```python
from build123d import *

# Parameters (mm, degrees)
BASE_FLANGE1_DEPTH           = 0.91186
F_2_5MM_DOWEL_HOLE1_D        = 2.5
EDGE_FLANGE1_STRIP_W         = 6.18744
EDGE_FLANGE1_STRIP_H         = 0.91186
EDGE_FLANGE1_STRIP_CUT_DEPTH = 82.55
EDGE_FLANGE1_DEPTH           = 82.55


# Sheet-metal steps are written as plain solids
with BuildPart() as part:
    # Sketch1 → Base-Flange1 (new body)
    with BuildSketch(Plane(origin=(0, 0, 0), x_dir=(1, 0, 0), z_dir=(0, 1, 0))):
        Polygon((0, -24.82463), (0, -48.018817445), (12.7, -48.018817445), (12.7, -37.52463), (69.85, -37.52463), (69.85, -48.018817445), (82.55, -48.018817445), (82.55, -24.82463), align=None)
    extrude(amount=-BASE_FLANGE1_DEPTH)

    # Ø2.5mm Dowel Hole1 (through all)
    with Locations(Plane(origin=(0, -0.91186, 0), x_dir=(-1, 0, 0), z_dir=(0, -1, 0))):
        with Locations((-65.76314, -27.56213), (-16.78686, -27.56213)):
            Hole(F_2_5MM_DOWEL_HOLE1_D / 2)

    # Edge-Flange1 strip (across the edge) → Edge-Flange1 strip cut (cut)
    with BuildSketch(Plane(origin=(82.55, 0, 24.82463), x_dir=(0, 0, 1), z_dir=(-1, 0, 0))):
        with Locations((-1.82372, -0.45593)):
            Rectangle(EDGE_FLANGE1_STRIP_W, EDGE_FLANGE1_STRIP_H)
    extrude(amount=EDGE_FLANGE1_STRIP_CUT_DEPTH, mode=Mode.SUBTRACT)

    # Edge-Flange1 section (across the edge) → Edge-Flange1 (add)
    with BuildSketch(Plane(origin=(82.55, 0, 24.82463), x_dir=(0, 0, 1), z_dir=(-1, 0, 0))):
        with BuildLine():
            Line((-0.91186, 1.27), (-0.91186, 5.43814))
            Line((-0.91186, 5.43814), (0, 5.43814))
            Line((0, 5.43814), (0, 1.27))
            ThreePointArc((0, 1.27), (0.371974388, 0.371974388), (1.27, 0))
            Line((1.27, 0), (1.27, -0.91186))
            ThreePointArc((1.27, -0.91186), (-0.272808002, -0.272808002), (-0.91186, 1.27))
        make_face()
    extrude(amount=EDGE_FLANGE1_DEPTH)


solid = part.part
```
Input: part model. Units: mm. Frame: model coordinates. A direction names the side the tool comes from. Give positions to 0.01 mm unless a question says otherwise; leave off trailing zeros. Order: outer loops, then holes, each group sorted by start corner. A loop starts at its lowest first (then second) coordinate and runs counter-clockwise, first axis right, second up. Notation, with made-up numbers: (18, 20.25) - (46, 20.25) arc R20 ccw to (46, 32.25) - close; hole circle Ø7 at (77, -14). An arc over 180 degrees is marked (long way). Put each result on its own line as item: value.
Item 1: Access query for faces 4 (the flat face through (41, 0, 34)), 5 (the flat face through (82.55, -0.3, 34.2)). Directions: +Z, -Z, +X, -X, +Y, -Y. A direction counts if a zero-diameter tool reaches every point of the face in a straight line with its end or side. Return the directions, or none.
Found:
face 4: +Z, +X, -X, +Y
face 5: +Z, -Z, +X, +Y, -Y
Item 2: Contact query for flat-ended pins moving along their axis: pin 1 (1.3 mm diameter, centred on x = 56, y = 3.5, fed in from +Z); pin 2 (2 mm diameter, centred on x = 65.76, z = 27.56, fed in from -Y); pin 3 (3 mm diameter, centred on x = 16.79, z = 27.56, fed in from +Y); pin 4 (0.5 mm diameter, centred on x = 30, y = -0.5, fed in from +Z). Output: stop coordinate, or through.
Found:
pin 1: stops at z = 24.82
pin 2: passes through
pin 3: stops at y = 0
pin 4: stops at z = 37.52
Item 3: Section query D-D, the plane z = 35.25. Return loops of the section in (x, y).
Found:
outline: (0, -0.91) - (82.55, -0.91) - (82.55, 0) - (0, 0) - close
Item 4: Ray query, L1, parallel to Z at x = 28, y = 4; L2, parallel to X at y = -0.5, z = 44.5; L3, parallel to Y at x = 76, z = 26.25. Return the intervals inside material, ascending. Write a range as from..to.
Found:
L1: z = 23.91..24.82
L2: x = 0..12.7, 69.85..82.55
L3: y = -0.91..0
Item 5: Section query A-A, the plane z = 42. Return loops of the section in (x, y), then the cut area to 3 significant figures.
Found:
outline: (0, -0.91) - (12.7, -0.91) - (12.7, 0) - (0, 0) - close; (69.85, -0.91) - (82.55, -0.91) - (82.55, 0) - (69.85, 0) - close
area: 23.2 mm^2
Item 6: Section query B-B, the plane x = 76.5. Return loops of the section in (y, z).
Found:
outline: (-0.91, 26.09) arc R2.18 ccw to (1.27, 23.91) - (5.44, 23.91) - (5.44, 24.82) - (1.27, 24.82) arc R1.27 cw to (0, 26.09) - (0, 48.02) - (-0.91, 48.02) - close
Item 7: Draft query along Z for faces 1 (the flat face through (41, -0.912, 34)), 2 (the cylindrical face through (15.795, -0.45, 28.323)), 3 (the flat face through (42, 3, 24.825)). Return one class per face: +Z half, -Z half, draft (parallel to the pull), parting line (faces both ways), or undercut.
Found:
face 1: draft
face 2: undercut
face 3: +Z half
Item 8: Section query C-C, the plane y = 3. Return loops of the section in (x, z), then the cut area to 3 significant figures.
Found:
outline: (0, 23.91) - (82.55, 23.91) - (82.55, 24.82) - (0, 24.82) - close
area: 75.3 mm^2
